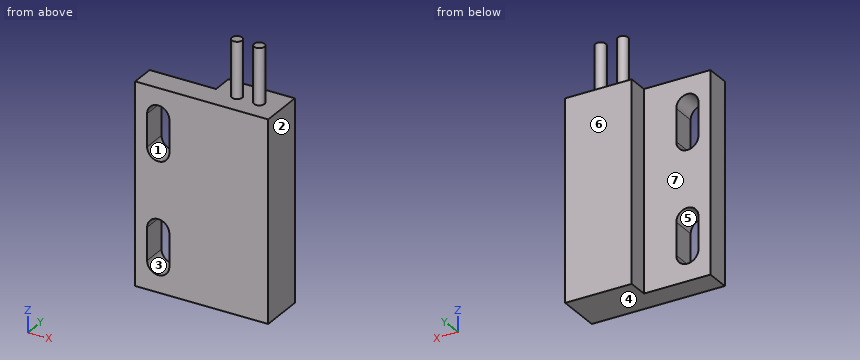
Autodesk Inventor part; units mm, degrees
ref_plane "YZ Plane" through (0, 0, 0) normal (1, 0, 0) x (0, 1, 0)
ref_plane "XZ Plane" through (0, 0, 0) normal (0, 1, 0) x (-1, 0, 0)
ref_plane "XY Plane" through (0, 0, 0) normal (0, 0, 1) x (1, 0, 0)
sketch "Sketch1" plane through (0, 0, 0) normal (0, 1, 0) x (-1, 0, 0)
  line L0 (0, 0) -> (19.05, 0)
  line L1 (19.05, 0) -> (19.05, -28.57)
  line L2 (19.05, -28.57) -> (0, -28.57)
  line L3 (0, -28.57) -> (0, 0)
  dimension "d0" = 19.05
  dimension "d1" = 28.57
extrude "Extrusion1" add sketch "Sketch1" along normal blind 3.43
sketch "Sketch2" plane through (0, 3.43, 0) normal (0, 1, 0) x (1, 0, 0)
  line L0 (0, 28.57) -> (-19.05, 28.57)
  line L1 (0, 0) -> (-9.53, 0)
  line L2 (-9.53, 0) -> (-9.53, 28.57)
  line L3 (-9.53, 28.57) -> (0, 28.57)
  line L4 (0, 28.57) -> (0, 0)
  dimension "d4" = 9.53
extrude "Extrusion2" add sketch "Sketch2" along normal blind 2.92
sketch "Sketch3" plane through (0, 6.35, 0) normal (0, 1, 0) x (1, 0, 0)
  line L0 (-15.75, 4.02) -> (-15.75, 8.66) construction
  line L1 (-14.16, 4.02) -> (-14.16, 8.66)
  line L2 (-17.34, 8.66) -> (-17.34, 4.02)
  arc A0 (-17.34, 4.02) -> (-14.16, 4.02) centre (-15.75, 4.02) ccw
  arc A1 (-14.16, 8.66) -> (-17.34, 8.66) centre (-15.75, 8.66) ccw
  line L3 (-19.05, 28.57) -> (-19.05, 0)
  line L4 (-15.75, 19.9) -> (-15.75, 24.54) construction
  line L5 (-14.16, 19.9) -> (-14.16, 24.54)
  line L6 (-17.34, 24.54) -> (-17.34, 19.9)
  arc A2 (-17.34, 19.9) -> (-14.16, 19.9) centre (-15.75, 19.9) ccw
  arc A3 (-14.16, 24.54) -> (-17.34, 24.54) centre (-15.75, 24.54) ccw
  line L7 (0, 28.57) -> (-9.53, 28.57)
  point P0 (0, 0)
  point P1 (-15.75, 6.34)
  point P2 (-15.75, 22.22)
  dimension "d7" = 4.64
  dimension "d8" = 3.18
  dimension "d9" = 3.3
  dimension "d10" = 4.64
  dimension "d11" = 3.18
  dimension "d12" = 15.88
  dimension "d13" = 6.35
extrude "Extrusion3" cut sketch "Sketch3" against normal through all
sketch "Sketch4" plane through (-19.05, 0, 0) normal (0, 0, 1) x (1, 0, 0)
  line L0 (9.52, 6.35) -> (19.05, 6.35)
  line L1 (9.52, 6.35) -> (12.69, 6.35)
  line L2 (12.69, 6.35) -> (12.69, 0)
  line L3 (0, 0) -> (19.05, 0)
  line L4 (19.05, 0) -> (19.05, 6.35)
  line L5 (19.05, 6.35) -> (15.87, 6.35)
  line L6 (15.87, 6.35) -> (15.87, 0)
  circle A0 centre (12.69, 3.175) radius 0.75
  circle A1 centre (15.87, 3.175) radius 0.75
  dimension "d20" = 3.17
  dimension "d21" = 3.18
  dimension "d24" = 1.5
  dimension "d25" = 1.5
extrude "Extrusion4" add sketch "Sketch4" along normal blind 8 contours A0 L2 | L2 A0 | A1 L6 | L6 A1
properties part number "59145_Sensor"
Here's how the part is built. I have some questions about the finished solid (model axes, mm). Face numbers are marked on the shaded views. A direction names the side the tool comes from. Round coordinates to 2 decimals unless told otherwise and drop trailing zeros. Order: outer loops, then holes, each group sorted by start corner. A loop starts at its lowest first (then second) coordinate and runs counter-clockwise, first axis right, second up. Notation, with made-up numbers: M 64.25,0.5 L 93.25,0.5 A25 ccw 93.25,23.5 Z; hole C 28,32 d10. An arc over 180 degrees is marked long. Return JSON: item names as keys, results as strings. Group by question number.
1. If we section it at D-D on z = -15.5: List the corners of the cut face in (x, y) for me, then the cut area to 3 significant figures.
2. If we section it at A-A on z = -22: List the corners of the cut face in (x, y) for me.
3. On a 3-axis mill with a long thin cutter (end or side, diameter ignored), from which of +Z, -Z, +X, -X, +Y, -Y can I reach the whole of each face in a straight line? I mean the marked faces 5, 6 and 7. Say none if no direction works.
4. I'm going to push flat-ended pins straight in: pin 1 Ø3 at (y, z) = (5, -11.5) entering from -X; pin 2 Ø7.5 at (x, z) = (-12, -20.5) entering from +Y; pin 3 Ø1 at (x, y) = (-8.5, 1.5) entering from +Z. Where does each tip first touch, or does it pass through?
5. If we mould it in two halves opening along Z, with no side actions, what happens to the marked faces 1, 2, 3 and 4? For each: pulls with the +Z half, pulls with the -Z half, needs draft (parallel to the pull), parting line crosses it, or undercut.
6. If we section it at C-C on x = -6.36: List the corners of the cut face in (y, z) for me (3 decimals).
7. Please list where these lines run through material, in increasing order: probe 1 along X at (y, z) = (0.5, -6.5); probe 2 along Y at (x, z) = (-14.75, -12); probe 3 along Z at (x, y) = (-5, 1.75).
8. If we section it at B-B on y = 1: List the corners of the cut face in (x, z) for me, then the cut area to 3 significant figures.
Reply:
{
 "1": {"outline": "M -19.05,0 L 0,0 L 0,6.35 L -9.53,6.35 L -9.53,3.43 L -19.05,3.43 Z", "area": "93.2 mm^2"},
 "2": {"outline": "M -19.05,0 L -17.34,0 L -17.34,3.43 L -19.05,3.43 Z; M -14.16,0 L 0,0 L 0,6.35 L -9.53,6.35 L -9.53,3.43 L -14.16,3.43 Z"},
 "3": {"face 5": "+Y, -Y", "face 6": "+Z, -Z, +X, -X, +Y", "face 7": "+Z, -Z, -X, +Y"},
 "4": {"pin 1": "x = -9.53", "pin 2": "y = 6.35", "pin 3": "z = 0"},
 "5": {"face 1": "undercut", "face 2": "needs draft", "face 3": "undercut", "face 4": "pulls with the -Z half"},
 "6": {"outline": "M 0,-28.57 L 6.35,-28.57 L 6.35,0 L 3.925,0 L 3.925,8 L 2.425,8 L 2.425,0 L 0,0 Z"},
 "7": {"probe 1": "-19.05 to -17.34, -14.16 to 0", "probe 2": "0 to 3.43", "probe 3": "-28.57 to 0"},
 "8": {"outline": "M -19.05,-28.57 L 0,-28.57 L 0,0 L -19.05,0 Z; hole M -17.34,-24.54 A1.59 ccw -14.16,-24.54 L -14.16,-19.9 A1.59 ccw -17.34,-19.9 Z; hole M -17.34,-8.66 A1.59 ccw -14.16,-8.66 L -14.16,-4.02 A1.59 ccw -17.34,-4.02 Z", "area": "499 mm^2"}
}
